```python
from build123d import *

# Parameters (mm, degrees)
BOSS_EXTRUDE1_DEPTH   = 3
SKETCH2_W             = 3
SKETCH2_H             = 25
BOSS_EXTRUDE2_DEPTH   = 30
CUT_EXTRUDE2_DEPTH    = 3
F_8_0MM_DOWEL_HOLE1_D = 8
F_8_0MM_DOWEL_HOLE2_D = 8
F_3_0MM_DOWEL_HOLE1_D = 3
F_3_0MM_DOWEL_HOLE2_D = 3
FILLET1_R             = 0.5


with BuildPart() as part:
    # Sketch1 → Boss-Extrude1 (new body)
    with BuildSketch(Plane(origin=(0, 0, 0), x_dir=(1, 0, 0), z_dir=(0, 1, 0))):
        with BuildLine():
            Line((-5, 12.5), (17.5, 12.5))
            Line((17.5, 12.5), (17.5, -12.5))
            Line((17.5, -12.5), (-5, -12.5))
            ThreePointArc((-5, -12.5), (-17.5, 0), (-5, 12.5))
        make_face()
    extrude(amount=BOSS_EXTRUDE1_DEPTH)

    # Sketch2 → Boss-Extrude2 (add)
    with BuildSketch(Plane(origin=(0, 3, 0), x_dir=(1, 0, 0), z_dir=(0, 1, 0))):
        with Locations((16, 0)):
            Rectangle(SKETCH2_W, SKETCH2_H)
    extrude(amount=BOSS_EXTRUDE2_DEPTH)

    # Sketch3 → Cut-Extrude2 (cut)
    with BuildSketch(Plane(origin=(17.5, 0, 0), x_dir=(0, 0, -1), z_dir=(1, 0, 0))):
        with BuildLine():
            Line((0, 33), (-12.5, 33))
            Line((-12.5, 33), (-12.5, 20.5))
            ThreePointArc((-12.5, 20.5), (-8.838834765, 29.338834765), (0, 33))
        make_face()
        with BuildLine():
            Line((12.5, 33), (0, 33))
            ThreePointArc((0, 33), (8.838834765, 29.338834765), (12.5, 20.5))
            Line((12.5, 20.5), (12.5, 33))
        make_face()
    extrude(amount=-CUT_EXTRUDE2_DEPTH, mode=Mode.SUBTRACT)

    # Ø8.0mm Dowel Hole1 (through all)
    with Locations(Plane(origin=(17.5, 0, 0), x_dir=(0, 0, -1), z_dir=(1, 0, 0))):
        with Locations((0, 20.5)):
            Hole(F_8_0MM_DOWEL_HOLE1_D / 2)

    # Ø8.0mm Dowel Hole2 (through all)
    with Locations(Plane(origin=(0, 3, 0), x_dir=(1, 0, 0), z_dir=(0, 1, 0))):
        with Locations((-5, 0)):
            Hole(F_8_0MM_DOWEL_HOLE2_D / 2)

    # Ø3.0mm Dowel Hole1 (through all)
    with Locations(Plane(origin=(17.5, 0, 0), x_dir=(0, 0, -1), z_dir=(1, 0, 0))):
        with Locations((0, 27.5), (7, 20.5), (0, 13.5), (-7, 20.5), (0, 20.5)):
            Hole(F_3_0MM_DOWEL_HOLE1_D / 2)

    # Ø3.0mm Dowel Hole2 (through all)
    with Locations(Plane(origin=(0, 3, 0), x_dir=(1, 0, 0), z_dir=(0, 1, 0))):
        with Locations((-12, 0), (-5, 7), (2, 0), (-5, -7), (-5, 0)):
            Hole(F_3_0MM_DOWEL_HOLE2_D / 2)

    # Fillet1
    fillet1_edges = [part.edges().sort_by_distance(p)[0] for p in [
        (4.75, 3, -12.5),
        (14.5, 11.75, 12.5),
        (17.5, 10.25, 12.5),
        (17.5, 33, 0),
        (14.5, 33, 0),
        (14.5, 11.75, -12.5),
        (17.5, 10.25, -12.5),
        (-17.5, 3, 0),
        (6.25, 0, -12.5),
        (6.25, 0, 12.5),
        (-17.5, 0, 0),
        (4.75, 3, 12.5),
    ]]
    fillet(fillet1_edges, radius=FILLET1_R)


solid = part.part
```
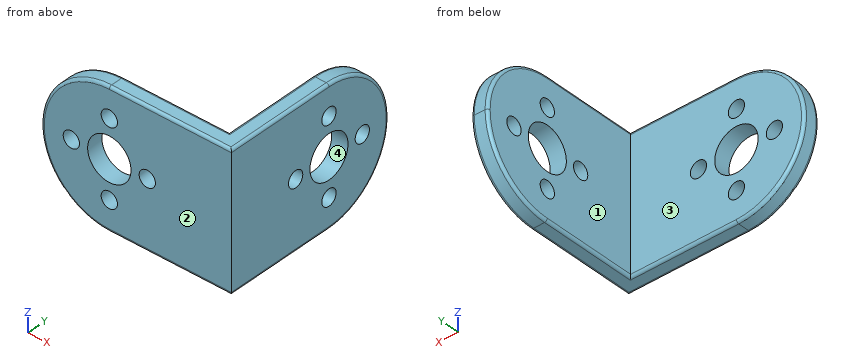
Work out the finished part from the listing and answer in its coordinate system (mm). Face numbers are marked on the shaded views. A direction names the side the tool comes from. Coordinates: 2 decimals unless noted, no trailing zeros. Loops run counter-clockwise (first coordinate to the right, second up) from the corner with the lowest first, then second, coordinate; pieces in that order, holes last. Notation, with made-up numbers: (-22.75, -0.5) - (29.25, -0.5) arc R26 cw to (29.25, 14.5) - close; hole circle Ø3 at (-9, 18). An arc over 180 degrees is marked (long way). Use a Markdown table: item, result.
Item 1: Find section C-C, the plane z = -7.5. State how many separate pieces and enclosed holes the cut face has, and give its area (3 significant figures).
Evaluation:
| item | result |
|---|---|
| separate pieces | 3 |
| enclosed holes | 0 |
| area | 163 mm2 |
Item 2: The mould has two halves that part along Z. Classify the marked faces 3 and 4: +Z half, -Z half, draft (parallel to the pull), parting line (faces both ways), or undercut.
Evaluation:
| item | result |
|---|---|
| face 3 | draft |
| face 4 | undercut |
Item 3: For the marked faces 1 and 2, determine the directions among +Z, -Z, +X, -X, +Y, -Y from which every point of the face is accessible in a straight line to the end or side of a thin tool.
Evaluation:
| item | result |
|---|---|
| face 1 | +Z, -Z, -X, +Y |
| face 2 | +Z, -Z, +X, -X, -Y |
Item 4: Find section B-B, the plane x = -0.5. Determine the outline of the cut face in (y, z).
Evaluation:
| item | result |
|---|---|
| outline | (0, -12) arc R0.5 ccw to (0.5, -12.5) - (2.5, -12.5) arc R0.5 ccw to (3, -12) - (3, 12) arc R0.5 ccw to (2.5, 12.5) - (0.5, 12.5) arc R0.5 ccw to (0, 12) - close |
Item 5: Consider probe 1 along Y at (x, z) = (15.65, 0); probe 2 along Z at (x, y) = (2, 1.1); probe 3 along X at (y, z) = (13, -6.25). Determine where each line is inside the solid, lowest interval first. Write a range as from..to.
Evaluation:
| item | result |
|---|---|
| probe 1 | y = 0..12, 15..16.5, 24.5..26, 29..33 |
| probe 2 | z = -12.5..-1.5, 1.5..12.5 |
| probe 3 | x = 14.5..17.5 |
Item 6: Find section A-A, the plane y = 10. Determine the outline of the cut face in (x, z).
Evaluation:
| item | result |
|---|---|
| outline | (14.5, -12) arc R0.5 ccw to (15, -12.5) - (17, -12.5) arc R0.5 ccw to (17.5, -12) - (17.5, 12) arc R0.5 ccw to (17, 12.5) - (15, 12.5) arc R0.5 ccw to (14.5, 12) - close |
Item 7: Given pin 1 Ø1.5 at (y, z) = (27, 1.5) entering from -X; pin 2 Ø13 at (x, z) = (-5, 0) entering from +Y; pin 3 Ø2.5 at (y, z) = (20.5, -7) entering from -X, each flat-ended and moving along its own axis, determine where each tip first touches the part or whether it passes through.
Evaluation:
| item | result |
|---|---|
| pin 1 | stops at x = 14.5 |
| pin 2 | stops at y = 3 |
| pin 3 | passes through |
